For this review, use the dimensioned drawing (mm, ordinates from the lowest corner) and the shaded views. A direction names the side the tool comes from. Give positions to 0.01 mm unless a question says otherwise; leave off trailing zeros. Write each loop counter-clockwise with the first axis right and the second up, starting at its lowest first coordinate (ties: lowest second). Pieces come first, ordered by that corner, then holes. Notation, with made-up numbers: M -40,70.5 L -6,70.5 A23 ccw -6,91.5 Z; hole C 46.25,31.5 d5. An arc over 180 degrees is marked long. One line per item, written item: value. Start each with the question number.
Item 1: Consider section B-B, the plane x = 8.5. Write out the cut boundary in (y, z).
Item 2: Clearance check with flat-ended pins moving along their axes: pin 1 Ø2 at (x, y) = (3.5, 3) entering from -Z; pin 2 Ø1 at (x, y) = (10.5, 1) entering from -Z. State where each tip first meets the part, or that it passes through.
Item 3: Consider section A-A, the plane y = 3.2. Write out the cut boundary in (x, z).
Item 4: Consider section D-D, the plane y = 2. Write out the cut boundary in (x, z).
Item 5: To check wall thickness, follow probe 1 along Z at (x, y) = (2.5, 1.65); probe 2 along X at (y, z) = (2.1, 6); probe 3 along X at (y, z) = (0.7, 1.25). State the ranges of each line that lie inside material, in increasing order.
Item 6: Tool access review of the marked faces 1 and 2: name each direction out of +Z, -Z, +X, -X, +Y, -Y from which nothing blocks a thin tool from reaching the whole face with its end or side.
Item 7: Consider section C-C, the plane z = 2. Write out the cut boundary in (x, y).
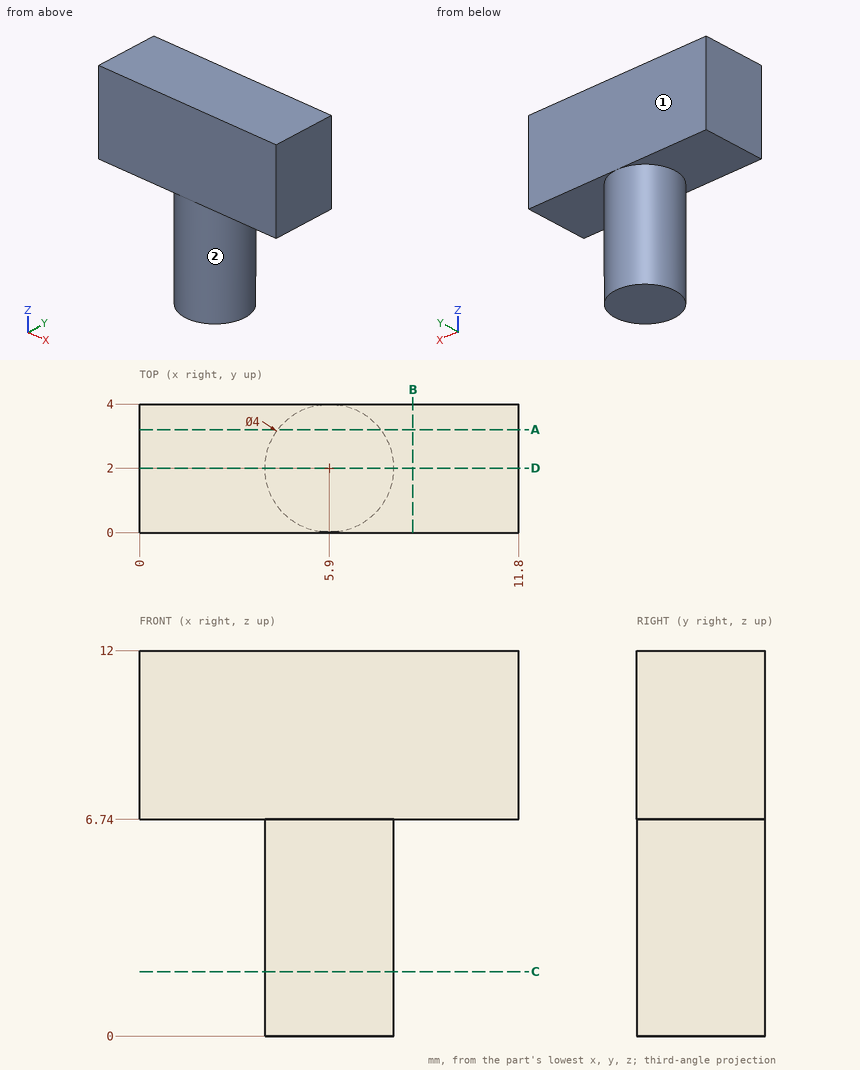
Model answer:
1. outline: M 0,6.74 L 4,6.74 L 4,12 L 0,12 Z
2. pin 1: stops at z = 0
2. pin 2: stops at z = 6.74
3. outline: M 0,6.74 L 4.3,6.74 L 4.3,0 L 7.5,0 L 7.5,6.74 L 11.8,6.74 L 11.8,12 L 0,12 Z
4. outline: M 0,6.74 L 3.9,6.74 L 3.9,0 L 7.9,0 L 7.9,6.74 L 11.8,6.74 L 11.8,12 L 0,12 Z
5. probe 1: z = 6.74 to 12
5. probe 2: x = 3.9 to 7.9
5. probe 3: x = 4.38 to 7.42
6. face 1: +Z, -Z, +X, -X, +Y
6. face 2: -Z
7. outline: C 5.9,2 d4
